```python
from build123d import *

# Parameters (mm, degrees)
SKETCH_1_R               = 44.7
EXTRUDE_1_DEPTH          = 3
SKETCH_1_5_R             = 1.5
CUT_EXTRUDE_1_DEPTH      = 73.5
SKETCH_1_6_R             = 2.1
CUT_EXTRUDE_2_DEPTH      = 42
PATTERN_CIRCULAR_1_COUNT = 6


with BuildPart() as part:
    # Sketch 1 → Extrude 1 (new body)
    with BuildSketch(Plane.XY):
        Circle(SKETCH_1_R)
    extrude(amount=EXTRUDE_1_DEPTH)

    # Sketch 1_5 → Cut-Extrude 1 (cut)
    with BuildSketch(Plane.XY):
        Circle(SKETCH_1_5_R)
    extrude(amount=CUT_EXTRUDE_1_DEPTH, mode=Mode.SUBTRACT)

    # Sketch 1_6 → Cut-Extrude 2 (cut)
    with BuildSketch(Plane.XY):
        with Locations((0, 39)):
            Circle(SKETCH_1_6_R)
    cut_extrude_2 = extrude(amount=CUT_EXTRUDE_2_DEPTH, mode=Mode.SUBTRACT)

    # Pattern Circular 1: Cut-Extrude 2 ×6 about axis
    pattern_circular_1_axis = Axis((0, 0, 0), (0, 0, 1))
    for i in range(1, PATTERN_CIRCULAR_1_COUNT):
        add(cut_extrude_2.rotate(pattern_circular_1_axis, i * 360 / PATTERN_CIRCULAR_1_COUNT), mode=Mode.SUBTRACT)


solid = part.part
```
Model file for the job. Use its own axes, mm. Round coordinates to 2 decimals unless told otherwise and drop trailing zeros. Write each loop counter-clockwise with the first axis right and the second up, starting at its lowest first coordinate (ties: lowest second). Pieces come first, ordered by that corner, then holes. Notation, with made-up numbers: (-13.75, 59) - (39.25, 59) arc R24 ccw to (39.25, 81) - close; hole circle Ø1 at (19, 74.5). An arc over 180 degrees is marked (long way). One line per item, written item: value.
(1) Cut at B-B, the plane y = 39. Give the cut face in (x, z), plus the area to 3 significant figures.
Values follow:
outline: (-21.84, 0) - (-2.1, 0) - (-2.1, 3) - (-21.84, 3) - close; (2.1, 0) - (21.84, 0) - (21.84, 3) - (2.1, 3) - close
area: 118 mm²
(2) Cut at A-A, the plane x = 0. Give the cut face in (y, z), plus the area to 3 significant figures.
Values follow:
outline: (-44.7, 0) - (-41.1, 0) - (-41.1, 3) - (-44.7, 3) - close; (-36.9, 0) - (-1.5, 0) - (-1.5, 3) - (-36.9, 3) - close; (1.5, 0) - (36.9, 0) - (36.9, 3) - (1.5, 3) - close; (41.1, 0) - (44.7, 0) - (44.7, 3) - (41.1, 3) - close
area: 234 mm²
(3) Drop flat-ended pins along their axis: P1, Ø1, axis at y = 29, z = 1.5, coming from the +X side; P2, Ø1, axis at x = -32.5, z = 0.5, coming from the +Y side. Give the stop position or say it passes through.
Values follow:
P1: stops at x = 34.44
P2: stops at y = 31.21
(4) Cut at C-C, the plane y = -19.5. Give the cut face in (x, z) (3 decimals).
Values follow:
outline: (-40.222, 0) - (-35.875, 0) - (-35.875, 3) - (-40.222, 3) - close; (-31.675, 0) - (31.675, 0) - (31.675, 3) - (-31.675, 3) - close; (35.875, 0) - (40.222, 0) - (40.222, 3) - (35.875, 3) - close
(5) Cut at D-D, the plane z = 1.65. Give the cut face in (x, y) (3 decimals).
Values follow:
outline: circle Ø89.4 at (0, 0); hole circle Ø4.2 at (-33.775, -19.5); hole circle Ø4.2 at (-33.775, 19.5); hole circle Ø4.2 at (0, -39); hole circle Ø4.2 at (0, 39); hole circle Ø3 at (0, 0); hole circle Ø4.2 at (33.775, -19.5); hole circle Ø4.2 at (33.775, 19.5)
(6) Two-plate mould, pull along Y, no slides. Class faces 1 (the cylindrical face through (-5.82, 44.32, 1.48)), 2 (the cylindrical face through (-34.23, -21.55, 1.48)), 3 (the flat face through (-1, -9, 3)): pulls with the +Y half, pulls with the -Y half, needs draft (parallel to the pull), parting line crosses it, or undercut.
Values follow:
face 1: parting line crosses it
face 2: undercut
face 3: needs draft
(7) Wall check: probe 1 along Y at (x, z) = (0, 0.7); probe 2 along Y at (x, z) = (-34.5, 1.8); probe 3 along X at (y, z) = (39, 1.1). Give the ranges that are in metal, low to high.
Values follow:
probe 1: y = -44.7 to -41.1, -36.9 to -1.5, 1.5 to 36.9, 41.1 to 44.7
probe 2: y = -28.42 to -21.47, -17.53 to 17.53, 21.47 to 28.42
probe 3: x = -21.84 to -2.1, 2.1 to 21.84
